Read the model definition and answer for the solid it produces. Units are mm, in the model's axes. A direction names the side the tool comes from. Coordinates: 2 decimals unless noted, no trailing zeros. Write each loop counter-clockwise with the first axis right and the second up, starting at its lowest first coordinate (ties: lowest second). Pieces come first, ordered by that corner, then holes.
Item 1: Determine the mould class of faces 4 (the face through (-1, -10, -69)), 5 (the face through (-1, 39, -10)), 6 (the face through (1, 33, -140)) for opening direction Y: released by +Y, released by -Y, zero draft, split by the parting line, or undercut.
Item 2: Each of these flat-tipped pins is pushed along its axis until it touches: P1, Ø1, axis at x = -17.5, z = -65, coming from the +Y side; P2, Ø4, axis at x = -22.5, y = 81, coming from the +Z side; P3, Ø1, axis at x = -6.5, z = -93, coming from the +Y side. Where does it stop, or does it pass through?
Item 3: Section A-A (x = 0) is taken. Give the vertices of the cut face in (y, z), then the cut area to 3 significant figures.
Item 4: Section C-C (z = -51) is taken. Give the vertices of the cut face in (x, y), then the cut area to 3 significant figures.
Item 5: Section D-D (z = -133.5) is taken. Give the vertices of the cut face in (x, y).
Item 6: A tool of negligible diameter and unlimited length cuts with its end or side. For faces 1 (the face through (-2.07, 88.765, -70.84)), 2 (the face through (-2.07, 88.765, 5.916)), 3 (the face through (-1, 0, -69)), from which of +Z, -Z, +X, -X, +Y, -Y can it reach the whole face along a straight path? Write none if from no direction.
Item 7: Section B-B (y = 40.5) is taken. Give the vertices of the cut face in (x, z), then the cut area to 3 significant figures.
Item 8: Straight lines are drawn through the part: probe 1 along Z at (x, y) = (14, 82); probe 2 along Y at (x, z) = (-13, -108); probe 3 along Y at (x, z) = (-16.5, -97). For each, find the intervals that lie inside material, in ascending order.
from build123d import *

# Parameters (mm, degrees)
EXTRUDE_1_DEPTH      = 12
EXTRUDE_1_DEPTH_BACK = 152
SKETCH_1_R           = 15.9
SKETCH_1_3_R         = 15.9
EXTRUDE_2_DEPTH      = 10
EXTRUDE_START        = 10
SKETCH_2_R           = 15.9
EXTRUDE_3_DEPTH      = 10
SKETCH_3_W           = 107
SKETCH_3_H           = 120
EXTRUDE_4_DEPTH      = 10


with BuildPart() as part:
    # 草图1 → 凸台-拉伸1 (new, two sides: drawn at the far end of the back side and taken through both)
    with BuildSketch(Plane.XY.offset(-EXTRUDE_1_DEPTH_BACK)):
        with Locations((0, 73)):
            Circle(SKETCH_1_R)
    extrude(amount=EXTRUDE_1_DEPTH + EXTRUDE_1_DEPTH_BACK)

    # 草图1<3> → 凸台-拉伸2 (add)
    with BuildSketch(Plane.XY):
        with BuildLine():
            Line((-53.5, 0), (-53.5, -10))
            Line((-53.5, -10), (53.5, -10))
            Line((53.5, -10), (53.5, 0))
            Line((53.5, 0), (23.462066716, 81.633158484))
            ThreePointArc((23.462066716, 81.633158484), (0, 98), (-23.462066716, 81.633158484))
            Line((-23.462066716, 81.633158484), (-53.5, 0))
        make_face()
        with Locations((0, 73)):
            Circle(SKETCH_1_3_R, mode=Mode.SUBTRACT)
    extrude(amount=-EXTRUDE_2_DEPTH)

    # 草图2 → 凸台-拉伸3 (add)
    with BuildSketch(Plane.XY.offset(-140).offset(EXTRUDE_START)):
        with BuildLine():
            Line((-53.5, 0), (-23.462066716, 81.633158484))
            ThreePointArc((-23.462066716, 81.633158484), (0, 98), (23.462066716, 81.633158484))
            Line((23.462066716, 81.633158484), (53.5, 0))
            Line((53.5, 0), (53.5, -10))
            Line((53.5, -10), (-53.5, -10))
            Line((-53.5, -10), (-53.5, 0))
        make_face()
        with Locations((0, 73)):
            Circle(SKETCH_2_R, mode=Mode.SUBTRACT)
    extrude(amount=-EXTRUDE_3_DEPTH)

    # 草图3 → 凸台-拉伸4 (add)
    with BuildSketch(Plane.XZ.offset(10)):
        with Locations((0, -70)):
            Rectangle(SKETCH_3_W, SKETCH_3_H)
    extrude(amount=-EXTRUDE_4_DEPTH)


solid = part.part
Established:
1. face 4: released by -Y
1. face 5: undercut
1. face 6: zero draft
2. P1: stops at y = 0
2. P2: stops at z = 0
2. P3: stops at y = 87.72
3. outline: (-10, -140) - (57.1, -140) - (57.1, -152) - (88.9, -152) - (88.9, -140) - (98, -140) - (98, -130) - (88.9, -130) - (88.9, -10) - (98, -10) - (98, 0) - (88.9, 0) - (88.9, 12) - (57.1, 12) - (57.1, 0) - (-10, 0) - close; hole (0, -130) - (57.1, -130) - (57.1, -10) - (0, -10) - close
3. area: 7,940 mm2
4. outline: (-53.5, -10) - (53.5, -10) - (53.5, 0) - (-53.5, 0) - close; circle Ø31.8 at (0, 73)
4. area: 1,860 mm2
5. outline: (-53.5, -10) - (53.5, -10) - (53.5, 0) - (23.46, 81.63) arc R25 ccw to (-23.46, 81.63) - (-53.5, 0) - close
6. face 1: none
6. face 2: +Z
6. face 3: +X, -X
7. outline: (-38.6, -140) - (38.6, -140) - (38.6, -130) - (-38.6, -130) - close; (-38.6, -10) - (38.6, -10) - (38.6, 0) - (-38.6, 0) - close
7. area: 1,540 mm2
8. probe 1: z = -140 to -130, -10 to 0
8. probe 2: y = -10 to 0, 63.85 to 82.15
8. probe 3: y = -10 to 0
